from build123d import *

# Parameters (mm, degrees)
F3_R      = 25.4
F3_R_2    = 24.8060859666
F4_DEPTH  = 41.275
F5_R      = 19.05
F6_DEPTH  = 41.276
F7_DEPTH  = 41.275
F8_DEPTH  = 41.276
F9_R      = 22.5
F9_R_2    = 19.05
F10_DEPTH = 17.78
F11_R     = 22.5
F11_R_2   = 19.05
F12_DEPTH = 17.78


with BuildPart() as f2:
    # F1 (on Front) → F2 (revolve)
    with BuildSketch(Plane.XZ):
        Polygon((-20.6375, 25.4), (0, 25.4), (20.6375, 25.4), (20.6375, 26.9582736391), (14.1049345586, 32.9880073607), (4.6889767244, 33.02), (0, 27.94), (-10.1817182737, 37.338), (-20.6375, 37.338), align=None)
    revolve(axis=Axis((0, 0, 0), (1, 0, 0)))

    # F3 (on face) → F4 (join, through all)
    with BuildSketch(Plane.YZ.offset(20.6375)):
        Circle(F3_R)
        Circle(F3_R_2, mode=Mode.SUBTRACT)
    extrude(amount=-F4_DEPTH)

    # F5 (on face) → F6 (cut, through all)
    with BuildSketch(Plane.YZ.offset(20.6375)):
        Circle(F5_R)
    extrude(amount=-F6_DEPTH, mode=Mode.SUBTRACT)

    # F3 (on face) → F7 (join, through all)
    with BuildSketch(Plane.YZ.offset(20.6375)):
        Circle(F3_R_2)
    extrude(amount=-F7_DEPTH)

    # F5 (on face) → F8 (cut, through all)
    with BuildSketch(Plane.YZ.offset(20.6375)):
        Circle(F5_R)
    extrude(amount=-F8_DEPTH, mode=Mode.SUBTRACT)

    # F9 (on face) → F10 (cut)
    with BuildSketch(Plane.YZ.offset(20.6375)):
        Circle(F9_R)
        Circle(F9_R_2, mode=Mode.SUBTRACT)
    extrude(amount=-F10_DEPTH, mode=Mode.SUBTRACT)

    # F11 (on face) → F12 (cut)
    with BuildSketch(Plane(origin=(-20.6375, 0, 0), x_dir=(0, -1, 0), z_dir=(-1, 0, 0))):
        Circle(F11_R)
        Circle(F11_R_2, mode=Mode.SUBTRACT)
    extrude(amount=-F12_DEPTH, mode=Mode.SUBTRACT)


solid = f2.part
Model file for the job. Use its own axes, mm. A direction names the side the tool comes from. Round coordinates to 2 decimals unless told otherwise and drop trailing zeros. Order: outer loops, then holes, each group sorted by start corner. A loop starts at its lowest first (then second) coordinate and runs counter-clockwise, first axis right, second up. Notation, with made-up numbers: M 86,-11 L 135,-11 A21 cw 135,7 Z; hole C 61.5,31 d2. An arc over 180 degrees is marked long. Write each question's results on one line, items separated by ' | '. Start each with the question number.
(1) Two-plate mould, pull along X, no slides. Class faces 4 (the face through (0.23, 17.15, -22.37)), 5 (the face through (-11.872, -10.382, -19.961)), 6 (the face through (20.638, -6, -22)), 7 (the face through (-2.857, 17, 10)): pulls with the +X half, pulls with the -X half, needs draft (parallel to the pull), parting line crosses it, or undercut.
(2) Which spindle directions (+Z, -Z, +X, -X, +Y, -Y) get a long thin tool onto all of the face, cutting with end or side? Do faces 1 (the face through (2.857, -17, 10)), 2 (the face through (-0.637, 27.85, -6.184)), 3 (the face through (0.04, -15.12, -11.59)). Say none if no direction does.
(3) Saw through at B-B, the plane x = 12.5. Give the cut face in (y, z).
(4) Saw through at A-A, the plane x = -6.5. Give the cut face in (y, z), then the cut area to 3 significant figures.
(5) Probe probe 1 along Z at (x, y) = (1, 0); probe 2 along Z at (x, y) = (7, -7.5); probe 3 along Y at (x, z) = (-13, -4). List the from-to ranges inside material, lowest first. Write a range as from..to.
(6) Drop flat-ended pins along their axis: pin 1 (2 mm diameter, centred on x = 13, z = -16, fed in from -Y); pin 2 (8 mm diameter, centred on x = -11.5, z = 29.5, fed in from -Y); pin 3 (5 mm diameter, centred on x = -13.5, y = -5.5, fed in from -Z). Give the stop position or say it passes through.
Established:
1) face 4: undercut | face 5: needs draft | face 6: pulls with the +X half | face 7: pulls with the -X half
2) face 1: +X | face 2: none | face 3: +X, -X
3) outline: C 0,0 d65.99; hole C 0,0 d45
4) outline: C 0,0 d67.88; hole C 0,0 d45 | area: 2,030 mm^2
5) probe 1: z = -29.02..-19.05, 19.05..29.02 | probe 2: z = -32.15..-21.21, 21.21..32.15 | probe 3: y = -37.12..-22.14, 22.14..37.12
6) pin 1: stops at y = -29.38 | pin 2: stops at y = -27.27 | pin 3: stops at z = -37.22
